Could you check a few things on this model? Use its own coordinates, in mm. A direction names the side the tool comes from. Round coordinates to 2 decimals unless told otherwise and drop trailing zeros. Loops run counter-clockwise (first coordinate to the right, second up) from the corner with the lowest first, then second, coordinate; pieces in that order, holes last. Notation, with made-up numbers: (6, 17.25) - (54, 17.25) arc R29 ccw to (54, 53.25) - close; hole circle Ø10 at (-22.75, 25.5). An arc over 180 degrees is marked (long way). Use one line per item in the form item = value.
```python
from build123d import *

# Parameters (mm, degrees)
SKETCH1_R           = 1.5875
BOSS_EXTRUDE1_DEPTH = 1.5875
FILLET1_R           = 0.4064
FILLET2_R           = 3.571875


with BuildPart() as part:
    # Sketch1 → Boss-Extrude1 (new body)
    with BuildSketch(Plane.XY):
        with BuildLine():
            Line((0, -1.5875), (52.3875, -1.5875))
            Line((52.3875, -1.5875), (52.3875, 0))
            Line((52.3875, 0), (57.15, 0))
            Line((57.15, 0), (57.15, -1.5875))
            Line((57.15, -1.5875), (63.5, -1.5875))
            Line((63.5, -1.5875), (63.5, 0))
            Line((63.5, 0), (68.2625, 0))
            Line((68.2625, 0), (68.2625, -1.5875))
            Line((68.2625, -1.5875), (74.6125, -1.5875))
            Line((74.6125, -1.5875), (74.6125, 6.35))
            Line((74.6125, 6.35), (68.2625, 6.35))
            Line((68.2625, 6.35), (50.472175754, 7.832527021))
            ThreePointArc((50.472175754, 7.832527021), (47.226754098, 9.508549174), (43.748686315, 8.392817807))
            Line((43.748686315, 8.392817807), (11.1125, 11.1125))
            ThreePointArc((11.1125, 11.1125), (7.744903955, 12.507403955), (6.35, 15.875))
            ThreePointArc((6.35, 15.875), (3.175, 19.05), (0, 15.875))
            Line((0, 15.875), (0, -1.5875))
        make_face()
        with Locations((3.175, 5.588)):
            Circle(SKETCH1_R, mode=Mode.SUBTRACT)
        with Locations((3.175, 13.462)):
            Circle(SKETCH1_R, mode=Mode.SUBTRACT)
        with Locations((11.90625, 4.7625)):
            Circle(SKETCH1_R, mode=Mode.SUBTRACT)
        with Locations((46.83125, 4.7625)):
            Circle(SKETCH1_R, mode=Mode.SUBTRACT)
    extrude(amount=BOSS_EXTRUDE1_DEPTH)

    # Fillet1
    fillet1_edges = [part.edges().sort_by_distance(p)[0] for p in [
        (68.2625, 6.35, 0.79375),
        (74.6125, 6.35, 0.79375),
        (74.6125, -1.5875, 0.79375),
        (68.2625, -1.5875, 0.79375),
        (68.2625, 0, 0.79375),
        (63.5, 0, 0.79375),
        (63.5, -1.5875, 0.79375),
        (57.15, -1.5875, 0.79375),
        (57.15, 0, 0.79375),
        (52.3875, 0, 0.79375),
        (52.3875, -1.5875, 0.79375),
        (0, -1.5875, 0.79375),
    ]]
    fillet(fillet1_edges, radius=FILLET1_R)

    # Fillet2
    fillet2_edges = [part.edges().sort_by_distance(p)[0] for p in [
        (43.748686315, 8.392817807, 0.79375),
        (50.472175754, 7.832527021, 0.79375),
    ]]
    fillet(fillet2_edges, radius=FILLET2_R)


solid = part.part
```
1. If we section it at D-D, the plane x = 23: Write out the boundary of the cut face in (y, z).
Solution:
outline = (-1.59, 0) - (10.12, 0) - (10.12, 1.59) - (-1.59, 1.59) - close
2. If we section it at C-C, the plane z = 0.4: Count the separate pieces of the cut face and the enclosed holes in it, plus the area to 3 significant figures.
Solution:
separate_pieces = 1
enclosed_holes = 4
area = 792 mm^2
3. We'd pull the mould along X, two halves only. Please class faces 1 (the face through (37, 4, 0)), 2 (the face through (66, 0, 1)), 3 (the face through (7.78, 12.47, 0.78)): +X half, -X half, draft (parallel to the pull), parting line (faces both ways), or undercut.
Solution:
face_1 = draft
face_2 = undercut
face_3 = +X half
4. If we section it at B-B, the plane y = 12.75: Write out the boundary of the cut face in (x, z).
Solution:
outline = (0, 0) - (1.76, 0) - (1.76, 1.59) - (0, 1.59) - close; (4.59, 0) - (7.52, 0) - (7.52, 1.59) - (4.59, 1.59) - close
5. Please list where these lines run through material, in increasing order: line 1 along Y through (x, z) = (3.5, 0.3); line 2 along X through (y, z) = (4.25, 0.9); line 3 along X through (y, z) = (4.5, 1.55).
Solution:
line_1 = -1.59 to 4.03, 7.14 to 11.91, 15.02 to 19.03
line_2 = 0 to 2.32, 4.03 to 10.4, 13.41 to 45.33, 48.33 to 74.61
line_3 = 0 to 2.02, 4.33 to 10.34, 13.47 to 45.27, 48.4 to 74.61
6. For P1, Ø0.5, axis at x = 54, z = 1, coming from the -Y side, with a flat end and sliding along its axis, tell me the tip position at first contact or that it passes through.
Solution:
P1 = 0
7. If we section it at A-A, the plane x = 12.5: Write out the boundary of the cut face in (y, z).
Solution:
outline = (-1.59, 0) - (3.29, 0) - (3.29, 1.59) - (-1.59, 1.59) - close; (6.23, 0) - (11, 0) - (11, 1.59) - (6.23, 1.59) - close
8. On a 3-axis mill with a long thin cutter (end or side, diameter ignored), from which of +Z, -Z, +X, -X, +Y, -Y can I reach the whole of each face in a straight line? I mean faces 4 (the face through (55, 0, 1)), 5 (the face through (45.245, 4.832, 0.783)), 6 (the face through (71, 6.35, 1)), 7 (the face through (27.027, 9.786, 0.783)). Say none if no direction works.
Solution:
face_4 = +Z, -Z, -Y
face_5 = +Z, -Z
face_6 = +Z, -Z, +X, +Y
face_7 = +Z, -Z, +Y
